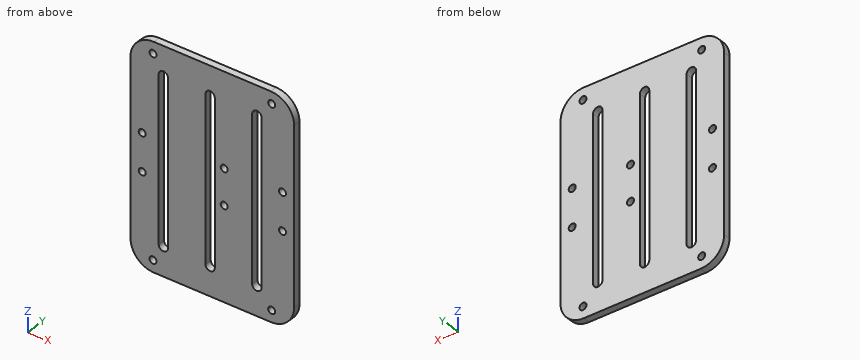
from build123d import *

# Parameters (mm, degrees)
SKETCH_1_R      = 1.5
EXTRUDE_1_DEPTH = 3


with BuildPart() as part:
    # 草图1 → 凸台-拉伸1 (new body)
    with BuildSketch(Plane(origin=(0, 0, 0), x_dir=(1, 0, 0), z_dir=(0, 1, 0))):
        with BuildLine():
            Line((-25, 47.42), (25, 47.42))
            ThreePointArc((25, 47.42), (32.071067812, 44.491067812), (35, 37.42))
            Line((35, 37.42), (35, -37.42))
            ThreePointArc((35, -37.42), (32.071067812, -44.491067812), (25, -47.42))
            Line((25, -47.42), (-25, -47.42))
            ThreePointArc((-25, -47.42), (-32.071067812, -44.491067812), (-35, -37.42))
            Line((-35, -37.42), (-35, 37.42))
            ThreePointArc((-35, 37.42), (-32.071067812, 44.491067812), (-25, 47.42))
        make_face()
        with Locations((-30, 8)):
            Circle(SKETCH_1_R, mode=Mode.SUBTRACT)
        with Locations((30, 8)):
            Circle(SKETCH_1_R, mode=Mode.SUBTRACT)
        with Locations((-30, -8)):
            Circle(SKETCH_1_R, mode=Mode.SUBTRACT)
        with Locations((30, -8)):
            Circle(SKETCH_1_R, mode=Mode.SUBTRACT)
        with Locations((-25.4, 42.42)):
            Circle(SKETCH_1_R, mode=Mode.SUBTRACT)
        with Locations((25.4, 42.42)):
            Circle(SKETCH_1_R, mode=Mode.SUBTRACT)
        with Locations((-25.4, -42.42)):
            Circle(SKETCH_1_R, mode=Mode.SUBTRACT)
        with Locations((25.4, -42.42)):
            Circle(SKETCH_1_R, mode=Mode.SUBTRACT)
        with Locations((5.08, -7.62)):
            Circle(SKETCH_1_R, mode=Mode.SUBTRACT)
        with Locations((5.08, 7.62)):
            Circle(SKETCH_1_R, mode=Mode.SUBTRACT)
        with BuildLine():
            Line((-22.95709571, -35), (-22.95709571, 35))
            ThreePointArc((-22.95709571, 35), (-20.95709571, 37), (-18.95709571, 35))
            Line((-18.95709571, 35), (-18.95709571, -35))
            ThreePointArc((-18.95709571, -35), (-20.95709571, -37), (-22.95709571, -35))
        make_face(mode=Mode.SUBTRACT)
        with BuildLine():
            Line((-2.95709571, -35), (-2.95709571, 35))
            ThreePointArc((-2.95709571, 35), (-0.95709571, 37), (1.04290429, 35))
            Line((1.04290429, 35), (1.04290429, -35))
            ThreePointArc((1.04290429, -35), (-0.95709571, -37), (-2.95709571, -35))
        make_face(mode=Mode.SUBTRACT)
        with BuildLine():
            Line((17.04290429, -35), (17.04290429, 35))
            ThreePointArc((17.04290429, 35), (19.04290429, 37), (21.04290429, 35))
            Line((21.04290429, 35), (21.04290429, -35))
            ThreePointArc((21.04290429, -35), (19.04290429, -37), (17.04290429, -35))
        make_face(mode=Mode.SUBTRACT)
    extrude(amount=EXTRUDE_1_DEPTH)


solid = part.part
Work out the finished part from the listing and answer in its coordinate system (mm). Coordinates: 2 decimals unless noted, no trailing zeros. Write each loop counter-clockwise with the first axis right and the second up, starting at its lowest first coordinate (ties: lowest second). Pieces come first, ordered by that corner, then holes. Notation, with made-up numbers: M 43.25,84 L 47.25,84 A30 cw 47.25,113 Z; hole C -22,-37 d7. An arc over 180 degrees is marked long. Answer as CSV lines item,"result". Start each with the question number.
Item 1: Section C-C on x = -1.5 is taken. Write down the section's boundary in (y, z), and give its area (3 significant figures).
Item 2: Section D-D on x = 29.5 is taken. Write down the section's boundary in (y, z).
Item 3: Section A-A on z = -15 is taken. Write down the section's boundary in (x, y).
Item 4: Consider L1, parallel to X at y = 2.1, z = -18.5; L2, parallel to Z at x = 30, y = 2.45; L3, parallel to Z at x = 5.5, y = 1.1. Determine where each line is inside the solid, lowest interval first.
Item 5: Section B-B on y = 2 is taken. Give the number of separate pieces and of enclosed holes in the cut face, and give its area (3 significant figures).
Checks:
1,outline,"M 0,-47.42 L 3,-47.42 L 3,-36.92 L 0,-36.92 Z; M 0,36.92 L 3,36.92 L 3,47.42 L 0,47.42 Z"
1,area,"63.0 mm²"
2,outline,"M 0,-46.35 L 3,-46.35 L 3,-9.41 L 0,-9.41 Z; M 0,-6.59 L 3,-6.59 L 3,6.59 L 0,6.59 Z; M 0,9.41 L 3,9.41 L 3,46.35 L 0,46.35 Z"
3,outline,"M -35,0 L -22.96,0 L -22.96,3 L -35,3 Z; M -18.96,0 L -2.96,0 L -2.96,3 L -18.96,3 Z; M 1.04,0 L 17.04,0 L 17.04,3 L 1.04,3 Z; M 21.04,0 L 35,0 L 35,3 L 21.04,3 Z"
4,L1,"x = -35 to -22.96, -18.96 to -2.96, 1.04 to 17.04, 21.04 to 35"
4,L2,"z = -46.08 to -9.5, -6.5 to 6.5, 9.5 to 46.08"
4,L3,"z = -47.42 to -9.06, -6.18 to 6.18, 9.06 to 47.42"
5,separate pieces,"1"
5,enclosed holes,"13"
5,area,"5,600 mm²"
